```python
from build123d import *

# Parameters (mm, degrees)
F0_W     = 14.351
F0_H     = 25.4
F0_R     = 1.5
F0_W_2   = 9.271
F0_H_2   = 11.176
F1_DEPTH = 6.35
F2_R     = 5.08
F3_R     = 1.27


with BuildPart() as f1:
    # F0 (on Front) → F1 (new body)
    with BuildSketch(Plane.XZ):
        with Locations((0, 7.62)):
            Rectangle(F0_W, F0_H)
        Circle(F0_R, mode=Mode.SUBTRACT)
        with Locations((0, 10.668)):
            Rectangle(F0_W_2, F0_H_2, mode=Mode.SUBTRACT)
    extrude(amount=F1_DEPTH)

    # F2
    f2_edges = [f1.edges().sort_by_distance(p)[0] for p in [
        (7.1755, -3.175, 20.32),
        (-7.1755, -3.175, 20.32),
    ]]
    fillet(f2_edges, radius=F2_R)

    # F3
    f3_edges = [f1.edges().sort_by_distance(p)[0] for p in [
        (7.1755, -3.175, -5.08),
        (-7.1755, -3.175, -5.08),
        (-4.6355, -3.175, 16.256),
        (4.6355, -3.175, 16.256),
        (-4.6355, -3.175, 5.08),
        (4.6355, -3.175, 5.08),
    ]]
    fillet(f3_edges, radius=F3_R)


solid = f1.part
```
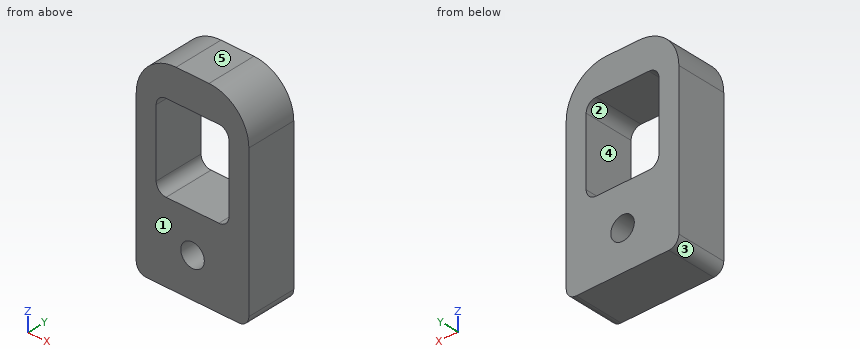
The model under review builds one solid part; all positions refer to its coordinate system, in mm. Face numbers are marked on the shaded views. A direction names the side the tool comes from. Coordinates: 2 decimals unless noted, no trailing zeros. Order: outer loops, then holes, each group sorted by start corner. A loop starts at its lowest first (then second) coordinate and runs counter-clockwise, first axis right, second up. Notation, with made-up numbers: (81, 89.25) -> (123, 89.25) arc R34 ccw to (123, 126.25) -> close; hole circle Ø10 at (14, -39.75). An arc over 180 degrees is marked (long way). Answer in a Markdown table with one row per item. Add a question column.
Item 1: We need section D-D on x = 3.75. Write out the cut boundary in (y, z).
Item 2: We need section B-B on z = 0. Write out the cut boundary in (x, y).
Item 3: To check wall thickness, follow probe 1 along Z at (x, y) = (0, -4); probe 2 along X at (y, z) = (-1, 15); probe 3 along Z at (x, y) = (1.75, -2.5). State the ranges of each line that lie inside material, in increasing order.
Item 4: We need section A-A on x = 0. Write out the cut boundary in (y, z).
Item 5: Mouldability with a two-part tool opening along X and no side actions: class the marked faces 1, 2 and 3 as +X half, -X half, draft (parallel to the pull), parting line (faces both ways), or undercut.
Item 6: We need section C-C on y = -5.25. Write out the cut boundary in (x, z), plus the area to 3 significant figures.
Item 7: Clearance check with a flat-ended pin moving along its axis: pin 1 (1 mm diameter, centred on x = -3, z = 4, fed in from +Y). State where the tip first meets the part, or that it passes through.
Item 8: Machinability: for the marked faces 4 and 5, which of the approach directions +Z, -Z, +X, -X, +Y, -Y give a long, thin tool a straight path to every point of the face, cutting with its end or side? Answer none if there is none.
Final values:
| question | item | result |
|---|---|---|
| 1 | outline | (-6.35, -5.08) -> (0, -5.08) -> (0, 5.14) -> (-6.35, 5.14) -> close; (-6.35, 16.2) -> (0, 16.2) -> (0, 20.04) -> (-6.35, 20.04) -> close |
| 2 | outline | (-7.18, -6.35) -> (-1.5, -6.35) -> (-1.5, 0) -> (-7.18, 0) -> close; (1.5, -6.35) -> (7.18, -6.35) -> (7.18, 0) -> (1.5, 0) -> close |
| 3 | probe 1 | z = -5.08 to -1.5, 1.5 to 5.08, 16.26 to 20.32 |
| 3 | probe 2 | x = -7.18 to -4.64, 4.64 to 7.18 |
| 3 | probe 3 | z = -5.08 to 5.08, 16.26 to 20.32 |
| 4 | outline | (-6.35, -5.08) -> (0, -5.08) -> (0, -1.5) -> (-6.35, -1.5) -> close; (-6.35, 1.5) -> (0, 1.5) -> (0, 5.08) -> (-6.35, 5.08) -> close; (-6.35, 16.26) -> (0, 16.26) -> (0, 20.32) -> (-6.35, 20.32) -> close |
| 5 | face 1 | draft |
| 5 | face 2 | undercut |
| 5 | face 3 | -X half |
| 6 | outline | (-7.18, -3.81) arc R1.27 ccw to (-5.91, -5.08) -> (5.91, -5.08) arc R1.27 ccw to (7.18, -3.81) -> (7.18, 15.24) arc R5.08 ccw to (2.1, 20.32) -> (-2.1, 20.32) arc R5.08 ccw to (-7.18, 15.24) -> close; hole (-4.64, 6.35) arc R1.27 ccw to (-3.37, 5.08) -> (3.37, 5.08) arc R1.27 ccw to (4.64, 6.35) -> (4.64, 14.99) arc R1.27 ccw to (3.37, 16.26) -> (-3.37, 16.26) arc R1.27 ccw to (-4.64, 14.99) -> close; hole circle Ø3 at (0, 0) |
| 6 | area | 243 mm2 |
| 7 | pin 1 | stops at y = 0 |
| 8 | face 4 | +Y, -Y |
| 8 | face 5 | +Z, +X, -X, +Y, -Y |
